from build123d import *

# Parameters (mm, degrees)
SK_HORN_PLATE_W   = 60
SK_HORN_PLATE_H   = 33.5
SK_HORN_PLATE_R   = 2
HORN_PLATE_DEPTH  = 4
SK_SERVO_PLATE_W  = 60
SK_SERVO_PLATE_H  = 53.36
SERVO_PLATE_DEPTH = 4


with BuildPart() as part:
    # SK_Horn_Plate → Horn_Plate (new body)
    with BuildSketch(Plane.XY.offset(3)):
        with Locations((10, -4.75)):
            Rectangle(SK_HORN_PLATE_W, SK_HORN_PLATE_H)
        Circle(SK_HORN_PLATE_R, mode=Mode.SUBTRACT)
    extrude(amount=HORN_PLATE_DEPTH)

    # SK_Servo_Plate → Servo_Plate (add)
    with BuildSketch(Plane(origin=(0, -21.5, 0), x_dir=(1, 0, 0), z_dir=(0, 1, 0))):
        with Locations((10, -29.68)):
            Rectangle(SK_SERVO_PLATE_W, SK_SERVO_PLATE_H)
    extrude(amount=SERVO_PLATE_DEPTH)


solid = part.part
The listing builds one solid part. Answer for the finished solid, in the listing's coordinates (mm). A direction names the side the tool comes from. Round coordinates to 2 decimals unless told otherwise and drop trailing zeros. Write each loop counter-clockwise with the first axis right and the second up, starting at its lowest first coordinate (ties: lowest second). Pieces come first, ordered by that corner, then holes. Notation, with made-up numbers: (77, -10.75) - (135, -10.75) arc R19 cw to (135, 26.25) - close; hole circle Ø6 at (-10.5, -12.5). An arc over 180 degrees is marked (long way). Use one line per item in the form item = value. Start each with the question number.
Item 1: A cutting plane is placed at A-A (x = 0). Write down the section's boundary in (y, z), plus the area to 3 significant figures.
Item 2: Flat-ended cylindrical pins translate along their axes: pin 1 Ø3.5 at (x, y) = (0, 0) entering from +Z; pin 2 Ø5 at (x, y) = (13, 5) entering from +Z; pin 3 Ø5 at (x, y) = (32, -16) entering from +Z. Find the tip coordinate at first contact, or state that the pin passes through.
Item 3: A cutting plane is placed at B-B (y = 0). Write down the section's boundary in (x, z), plus the area to 3 significant figures.
Item 4: A tool of negligible diameter and unlimited length cuts with its end or side. For faces 1 (the flat face through (10, -17.5, 31)), 2 (the flat face through (-20, -18, 20)), from which of +Z, -Z, +X, -X, +Y, -Y can it reach the whole face along a straight path? Write none if from no direction.
Item 5: Determine the mould class of faces 3 (the flat face through (40, -18, 20)), 4 (the flat face through (10, -3, 7)), 5 (the cylindrical face through (0, -2, 5)) for opening direction X: +X half, -X half, draft (parallel to the pull), parting line (faces both ways), or undercut.
Item 6: Find the intervals of material crossed by line 1 (Y direction, x = 0, z = 4.15); line 2 (Y direction, x = 34, z = 25); line 3 (Z direction, x = -10, y = -13), in increasing order. Write a range as [from, to].
Item 7: A cutting plane is placed at C-C (x = 15.5). Write down the section's boundary in (y, z).
Item 8: A cutting plane is placed at D-D (z = 27.5). Write down the section's boundary in (x, y), plus the area to 3 significant figures.
The answers:
q1.outline = (-21.5, 3) - (-2, 3) - (-2, 7) - (-17.5, 7) - (-17.5, 56.36) - (-21.5, 56.36) - close; (2, 3) - (12, 3) - (12, 7) - (2, 7) - close
q1.area = 315 mm^2
q2.pin_1 = through
q2.pin_2 = 7
q2.pin_3 = 56.36
q3.outline = (-20, 3) - (-2, 3) - (-2, 7) - (-20, 7) - close; (2, 3) - (40, 3) - (40, 7) - (2, 7) - close
q3.area = 224 mm^2
q4.face_1 = +Z, +X, -X, +Y
q4.face_2 = +Z, -Z, -X, +Y, -Y
q5.face_3 = +X half
q5.face_4 = draft
q5.face_5 = undercut
q6.line_1 = [-21.5, -2], [2, 12]
q6.line_2 = [-21.5, -17.5]
q6.line_3 = [3, 7]
q7.outline = (-21.5, 3) - (12, 3) - (12, 7) - (-17.5, 7) - (-17.5, 56.36) - (-21.5, 56.36) - close
q8.outline = (-20, -21.5) - (40, -21.5) - (40, -17.5) - (-20, -17.5) - close
q8.area = 240 mm^2
